```python
from build123d import *

# Parameters (mm, degrees)
SKETCH1_R           = 10
BOSS_EXTRUDE1_DEPTH = 15
SKETCH2_R           = 9
SKETCH2_R_2         = 3
CUT_EXTRUDE1_DEPTH  = 0.5
SKETCH3_R           = 2
CUT_EXTRUDE2_DEPTH  = 3


with BuildPart() as part:
    # Sketch1 → Boss-Extrude1 (new body)
    with BuildSketch(Plane.XY):
        Circle(SKETCH1_R)
    extrude(amount=BOSS_EXTRUDE1_DEPTH)

    # Sketch2 → Cut-Extrude1 (cut)
    with BuildSketch(Plane.XY.offset(15)):
        Circle(SKETCH2_R)
        Circle(SKETCH2_R_2, mode=Mode.SUBTRACT)
    extrude(amount=-CUT_EXTRUDE1_DEPTH, mode=Mode.SUBTRACT)

    # Sketch3 → Cut-Extrude2 (cut)
    with BuildSketch(Plane(origin=(0, 0, 0), x_dir=(-1, 0, 0), z_dir=(0, 0, -1))):
        Circle(SKETCH3_R)
    extrude(amount=-CUT_EXTRUDE2_DEPTH, mode=Mode.SUBTRACT)


solid = part.part
```
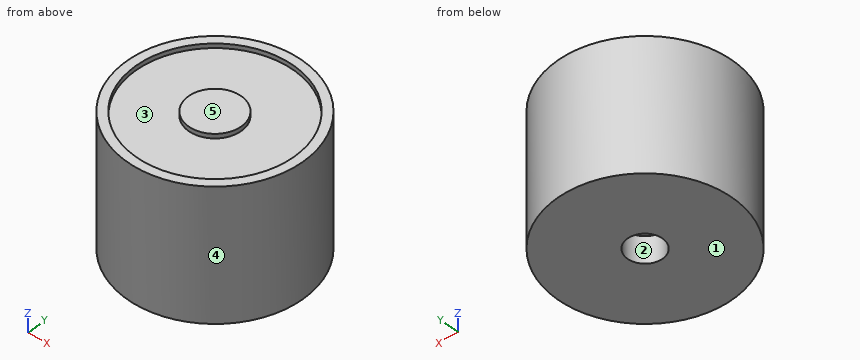
Could you check a few things on this model? Use its own coordinates, in mm. Face numbers are marked on the shaded views. A direction names the side the tool comes from. Give positions to 0.01 mm unless a question says otherwise; leave off trailing zeros. Order: outer loops, then holes, each group sorted by start corner. A loop starts at its lowest first (then second) coordinate and runs counter-clockwise, first axis right, second up.
Q1. Suppose I cut it at B-B, the plane x = -7. Write out the boundary of the cut face in (y, z).
Q2. If I drill on line 1 along Y through (x, z) = (0, 14.6); line 2 along Z through (x, y) = (1, 5.25); line 3 along Y through (x, z) = (-0.5, 0.75), over which ranges is the centre line in solid material (lowest first)?
Q3. Suppose I cut it at D-D, the plane y = 4.75. Write out the boundary of the cut face in (x, z).
Q4. I'm going to push flat-ended pins straight in: P1, Ø6, axis at y = 3.5, z = 12.5, coming from the -X side; P2, Ø1.5, axis at x = -3, y = -7, coming from the +Z side; P3, Ø2, axis at x = -0.5, y = 0.5, coming from the -Z side. Where does each tip first touch, or does it pass through?
Q5. We'd pull the mould along X, two halves only. Please class the marked faces 3, 4 and 5: +X half, -X half, draft (parallel to the pull), parting line (faces both ways), or undercut.
Q6. Suppose I cut it at C-C, the plane z = 6. Write out the boundary of the cut face in (x, y).
Q7. Suppose I cut it at A-A, the plane y = 0. Write out the boundary of the cut face in (x, z).
Q8. For the marked faces 1 and 2, which set-ups out of +Z, -Z, +X, -X, +Y, -Y let a thin tool reach every point of the face, with its end or its side?
Solution:
1. outline: (-7.14, 0) - (7.14, 0) - (7.14, 15) - (5.66, 15) - (5.66, 14.5) - (-5.66, 14.5) - (-5.66, 15) - (-7.14, 15) - close
2. line 1: y = -10 to -9, -3 to 3, 9 to 10
2. line 2: z = 0 to 14.5
2. line 3: y = -9.99 to -1.94, 1.94 to 9.99
3. outline: (-8.8, 0) - (8.8, 0) - (8.8, 15) - (7.64, 15) - (7.64, 14.5) - (-7.64, 14.5) - (-7.64, 15) - (-8.8, 15) - close
4. P1: stops at x = -9.99
4. P2: stops at z = 14.5
4. P3: stops at z = 3
5. face 3: undercut
5. face 4: parting line
5. face 5: draft
6. outline: circle Ø20 at (0, 0)
7. outline: (-10, 0) - (-2, 0) - (-2, 3) - (2, 3) - (2, 0) - (10, 0) - (10, 15) - (9, 15) - (9, 14.5) - (3, 14.5) - (3, 15) - (-3, 15) - (-3, 14.5) - (-9, 14.5) - (-9, 15) - (-10, 15) - close
8. face 1: -Z, +X, -X, +Y, -Y
8. face 2: -Z
